from build123d import *

# Parameters (mm, degrees)
SKETCH_1_W          = 35
SKETCH_1_H          = 40
SKETCH_1_R          = 1.5
EXTRUDE_1_DEPTH     = 4
SKETCH_2_W          = 40
SKETCH_2_H          = 18
EXTRUDE_2_DEPTH     = 4
SKETCH_3_W          = 40
SKETCH_3_H          = 4
EXTRUDE_3_DEPTH     = 12
CUT_EXTRUDE_1_REACH = 44.968
SKETCH_4_R          = 1.5
CHAMFER_1_SIZE      = 2


with BuildPart() as part:
    # 草图1 → 凸台-拉伸1 (new body)
    with BuildSketch(Plane(origin=(0, 0, 0), x_dir=(1, 0, 0), z_dir=(0, 1, 0))):
        Rectangle(SKETCH_1_W, SKETCH_1_H)
        with Locations(Location((12.5, 10, 0), (0, 0, 270))):
            Circle(SKETCH_1_R, mode=Mode.SUBTRACT)
        with Locations(Location((-12.5, 10, 0), (0, 0, 90))):
            Circle(SKETCH_1_R, mode=Mode.SUBTRACT)
        with Locations(Location((-12.5, -10, 0), (0, 0, 270))):
            Circle(SKETCH_1_R, mode=Mode.SUBTRACT)
        with Locations(Location((12.5, -10, 0), (0, 0, 90))):
            Circle(SKETCH_1_R, mode=Mode.SUBTRACT)
    extrude(amount=EXTRUDE_1_DEPTH)

    # 草图2 → 凸台-拉伸2 (add)
    with BuildSketch(Plane.ZY.offset(17.5)):
        with Locations((0, 9)):
            Rectangle(SKETCH_2_W, SKETCH_2_H)
    extrude(amount=EXTRUDE_2_DEPTH)

    # 草图3 → 凸台-拉伸3 (add)
    with BuildSketch(Plane.ZY.offset(21.5)):
        with Locations((0, 16)):
            Rectangle(SKETCH_3_W, SKETCH_3_H)
    extrude(amount=EXTRUDE_3_DEPTH)

    # 草图4 → 切除-拉伸1 (cut, up to next)
    with BuildSketch(Plane(origin=(0, 18, 0), x_dir=(1, 0, 0), z_dir=(0, 1, 0)), mode=Mode.PRIVATE) as cut_extrude_1_sk1:
        with Locations(Location((-27.5, 0, 0), (0, 0, 270))):
            Circle(SKETCH_4_R)
    cut_extrude_1_tool1 = extrude(cut_extrude_1_sk1.sketch, amount=-CUT_EXTRUDE_1_REACH, mode=Mode.PRIVATE) & part.part
    add(cut_extrude_1_tool1.solids().sort_by_distance((-27.5, 18, 0))[0], mode=Mode.SUBTRACT)

    # 倒角1
    chamfer_1_edges = [part.edges().sort_by_distance(p)[0] for p in [
        (-27.5, 18, -1.5),
    ]]
    chamfer(chamfer_1_edges, length=CHAMFER_1_SIZE)


solid = part.part
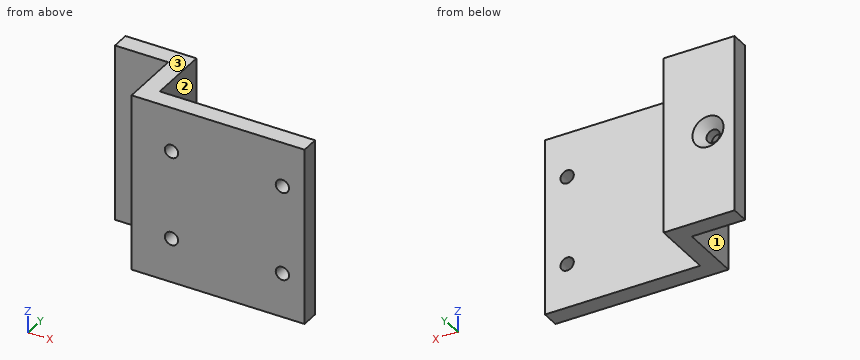
CAD build for the part. Positions are in the model's coordinates, mm. Face numbers are marked on the shaded views. A direction names the side the tool comes from. Round coordinates to 2 decimals unless told otherwise and drop trailing zeros. Order: outer loops, then holes, each group sorted by start corner. A loop starts at its lowest first (then second) coordinate and runs counter-clockwise, first axis right, second up. Notation, with made-up numbers: M 60,41 L 109,41 A30 ccw 109,78 Z; hole C 61,34.25 d11. An arc over 180 degrees is marked long. Use one line per item in the form item = value.
Q1. Saw through at C-C on x = -27.5. Give the cut face in (y, z), then the cut area to 3 significant figures.
Recorded:
outline = M 14,-20 L 18,-20 L 18,-3.5 L 16,-1.5 L 14,-1.5 Z; M 14,1.5 L 16,1.5 L 18,3.5 L 18,20 L 14,20 Z
area = 144 mm^2
Q2. Saw through at D-D on z = 0. Give the cut face in (x, y), then the cut area to 3 significant figures.
Recorded:
outline = M -33.5,14 L -29,14 L -29,16 L -31,18 L -33.5,18 Z; M -26,14 L -21.5,14 L -21.5,0 L 17.5,0 L 17.5,4 L -17.5,4 L -17.5,18 L -24,18 L -26,16 Z
area = 244 mm^2
Q3. Probe L1, parallel to X at y = 2.05, z = -10; L2, parallel to X at y = 15.05, z = 0; L3, parallel to X at y = 2, z = -7. List the from-to ranges inside material, lowest first.
Recorded:
L1 = -21.5 to -14, -11 to 11, 14 to 17.5
L2 = -33.5 to -29, -26 to -17.5
L3 = -21.5 to 17.5
Q4. Which spindle directions (+Z, -Z, +X, -X, +Y, -Y) get a long thin tool onto all of the face, cutting with end or side? Do the marked faces 1, 2 and 3. Say none if no direction does.
Recorded:
face_1 = +Z, -Z, -X, -Y
face_2 = +Z, -Z, +X, +Y
face_3 = +Z, +X, -X, +Y, -Y
Q5. Saw through at B-B on z = -10. Give the cut face in (x, y).
Recorded:
outline = M -33.5,14 L -21.5,14 L -21.5,0 L -14,0 L -14,4 L -17.5,4 L -17.5,18 L -33.5,18 Z; M -11,0 L 11,0 L 11,4 L -11,4 Z; M 14,0 L 17.5,0 L 17.5,4 L 14,4 Z
Q6. Flat gauge pins, fed straight in: P1, Ø1.5, axis at x = -5.5, z = 2, coming from the +Y side; P2, Ø4, axis at y = 9.5, z = -6.5, coming from the +X side; P3, Ø2.5, axis at x = -12.5, z = -10, coming from the -Y side; P4, Ø3.5, axis at x = -29, z = 8.5, coming from the -Y side. Where does each tip first touch, or does it go through?
Recorded:
P1 = 4
P2 = -17.5
P3 = through
P4 = 14
Q7. Saw through at A-A on x = 12.5. Give the cut face in (y, z), then the cut area to 3 significant figures.
Recorded:
outline = M 0,-20 L 4,-20 L 4,-11.5 L 0,-11.5 Z; M 0,-8.5 L 4,-8.5 L 4,8.5 L 0,8.5 Z; M 0,11.5 L 4,11.5 L 4,20 L 0,20 Z
area = 136 mm^2
